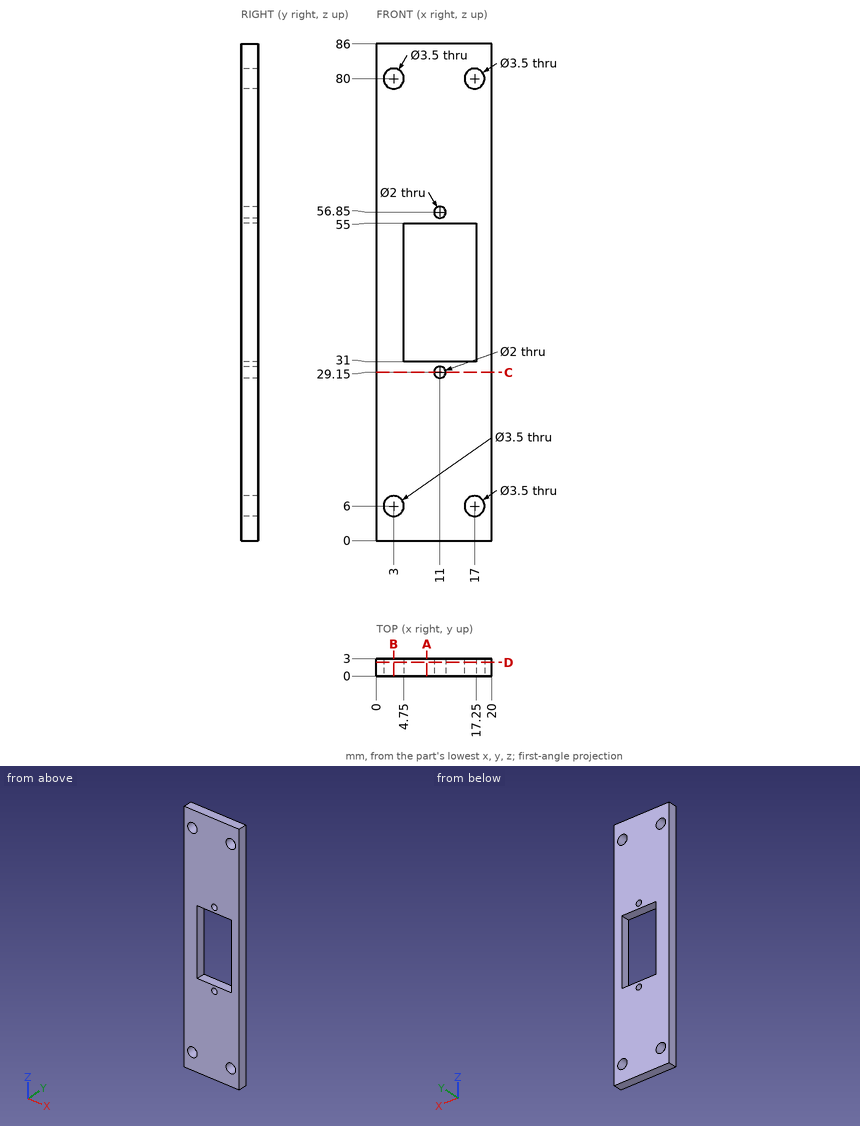
For this review, use the dimensioned drawing (mm, ordinates from the lowest corner) and the shaded views. Give positions to 0.01 mm unless a question says otherwise; leave off trailing zeros. Loops run counter-clockwise (first coordinate to the right, second up) from the corner with the lowest first, then second, coordinate; pieces in that order, holes last. Notation, with made-up numbers: (-33, -27.75) - (3, -27.75) arc R23 ccw to (3, -17.75) - close; hole circle Ø3 at (-30.5, 47). An arc over 180 degrees is marked (long way). Write each question's results on one line, items separated by ' | '.
(1) Take a section at D-D (y = 2.35). Give the boundary of the cut face in (x, z).
Conclusion:
outline: (0, 0) - (20, 0) - (20, 86) - (0, 86) - close; hole circle Ø3.5 at (3, 6); hole circle Ø3.5 at (3, 80); hole (4.75, 31) - (17.25, 31) - (17.25, 55) - (4.75, 55) - close; hole circle Ø2 at (11, 29.15); hole circle Ø2 at (11, 56.85); hole circle Ø3.5 at (17, 6); hole circle Ø3.5 at (17, 80)
(2) Take a section at C-C (z = 29.15). Give the boundary of the cut face in (x, y).
Conclusion:
outline: (0, 0) - (10, 0) - (10, 3) - (0, 3) - close; (12, 0) - (20, 0) - (20, 3) - (12, 3) - close
(3) Take a section at A-A (x = 8.75). Give the boundary of the cut face in (y, z), then the cut area to 3 significant figures.
Conclusion:
outline: (0, 0) - (3, 0) - (3, 31) - (0, 31) - close; (0, 55) - (3, 55) - (3, 86) - (0, 86) - close | area: 186 mm^2
(4) Take a section at B-B (x = 3). Give the boundary of the cut face in (y, z).
Conclusion:
outline: (0, 0) - (3, 0) - (3, 4.25) - (0, 4.25) - close; (0, 7.75) - (3, 7.75) - (3, 78.25) - (0, 78.25) - close; (0, 81.75) - (3, 81.75) - (3, 86) - (0, 86) - close
(5) For line 1 along Z through (x, y) = (17, 2); line 2 along Z through (x, y) = (11, 2.2); line 3 along X through (y, z) = (0.95, 6), list the stretches that pass through material, from the lowest coordinate up.
Conclusion:
line 1: 0 to 4.25, 7.75 to 31, 55 to 78.25, 81.75 to 86 | line 2: 0 to 28.15, 30.15 to 31, 55 to 55.85, 57.85 to 86 | line 3: 0 to 1.25, 4.75 to 15.25, 18.75 to 20
